Build history of the part. All positions in model axes, mm. Face numbers are marked on the shaded views. A direction names the side the tool comes from. Round coordinates to 2 decimals unless told otherwise and drop trailing zeros. Loops run counter-clockwise (first coordinate to the right, second up) from the corner with the lowest first, then second, coordinate; pieces in that order, holes last.
from build123d import *

# Parameters (mm, degrees)
SKETCH1_R                = 48
SKETCH1_R_2              = 5.25
BOSS_EXTRUDE1_DEPTH      = 9
SKETCH2_R                = 22.5
CUT_EXTRUDE1_DEPTH       = 3.4
SKETCH3_R                = 12
CUT_EXTRUDE2_DEPTH       = 6.6
BOSS_EXTRUDE2_DEPTH      = 17
BOSS_EXTRUDE2_DEPTH_BACK = 17
SKETCH5_R                = 12
CUT_EXTRUDE3_DEPTH       = 4.5
CUT_EXTRUDE3_DEPTH_BACK  = 4.5
CUT_EXTRUDE4_DEPTH       = 12.5
CUT_EXTRUDE4_DEPTH_BACK  = 85.5
SKETCH8_R                = 12
CUT_EXTRUDE5_DEPTH       = 12.5
CUT_EXTRUDE5_DEPTH_BACK  = 85.5


with BuildPart() as part:
    # Sketch1 → Boss-Extrude1 (new body)
    with BuildSketch(Plane(origin=(0, 0, 0), x_dir=(1, 0, 0), z_dir=(0, 1, 0))):
        Circle(SKETCH1_R)
        with Locations((0, 40)):
            Circle(SKETCH1_R_2, mode=Mode.SUBTRACT)
        with Locations((40, 0)):
            Circle(SKETCH1_R_2, mode=Mode.SUBTRACT)
        with Locations((0, -40)):
            Circle(SKETCH1_R_2, mode=Mode.SUBTRACT)
        with Locations((-40, 0)):
            Circle(SKETCH1_R_2, mode=Mode.SUBTRACT)
    extrude(amount=BOSS_EXTRUDE1_DEPTH)

    # Sketch2 → Cut-Extrude1 (cut)
    with BuildSketch(Plane(origin=(0, 9, 0), x_dir=(1, 0, 0), z_dir=(0, 1, 0))):
        Circle(SKETCH2_R)
    extrude(amount=-CUT_EXTRUDE1_DEPTH, mode=Mode.SUBTRACT)

    # Sketch3 → Cut-Extrude2 (cut, through all)
    with BuildSketch(Plane(origin=(0, 5.6, 0), x_dir=(1, 0, 0), z_dir=(0, 1, 0))):
        Circle(SKETCH3_R)
    extrude(amount=-CUT_EXTRUDE2_DEPTH, mode=Mode.SUBTRACT)

    # Sketch4 → Boss-Extrude2 (add, two sides)
    with BuildSketch(Plane.XY) as boss_extrude2_sk:
        with BuildLine():
            Line((-36.5, -66), (-36.5, -32))
            ThreePointArc((-36.5, -32), (-36.207106781, -31.292893219), (-35.5, -31))
            Line((-35.5, -31), (-35.5, -15))
            ThreePointArc((-35.5, -15), (-34.482827555, -7.237912652), (-31.5, 0))
            Line((-31.5, 0), (31.5, 0))
            ThreePointArc((31.5, 0), (34.482827555, -7.237912652), (35.5, -15))
            Line((35.5, -15), (35.5, -31))
            ThreePointArc((35.5, -31), (36.207106781, -31.292893219), (36.5, -32))
            Line((36.5, -32), (36.5, -66))
            ThreePointArc((36.5, -66), (36.207106781, -66.707106781), (35.5, -67))
            Line((35.5, -67), (19.5, -67))
            ThreePointArc((19.5, -67), (18.792893219, -66.707106781), (18.5, -66))
            Line((18.5, -66), (18.5, -12))
            ThreePointArc((18.5, -12), (16.156854249, -6.343145751), (10.5, -4))
            Line((10.5, -4), (-10.5, -4))
            ThreePointArc((-10.5, -4), (-16.156854249, -6.343145751), (-18.5, -12))
            Line((-18.5, -12), (-18.5, -66))
            ThreePointArc((-18.5, -66), (-18.792893219, -66.707106781), (-19.5, -67))
            Line((-19.5, -67), (-35.5, -67))
            ThreePointArc((-35.5, -67), (-36.207106781, -66.707106781), (-36.5, -66))
        make_face()
    extrude(amount=BOSS_EXTRUDE2_DEPTH)
    extrude(boss_extrude2_sk.sketch, amount=-BOSS_EXTRUDE2_DEPTH_BACK)

    # Sketch5 → Cut-Extrude3 (cut, two sides)
    with BuildSketch(Plane.XZ.offset(4)) as cut_extrude3_sk:
        Circle(SKETCH5_R)
    extrude(amount=CUT_EXTRUDE3_DEPTH, mode=Mode.SUBTRACT)
    extrude(cut_extrude3_sk.sketch, amount=-CUT_EXTRUDE3_DEPTH_BACK, mode=Mode.SUBTRACT)

    # Sketch7 → Cut-Extrude4 (cut, two sides)
    with BuildSketch(Plane.ZY.offset(36.5)) as cut_extrude4_sk:
        with BuildLine():
            Line((-17, 0), (-17, -49))
            ThreePointArc((-17, -49), (0, -66), (17, -49))
            Line((17, -49), (17, 0))
            Line((17, 0), (31.554606814, 0))
            Line((31.554606814, 0), (31.554606814, -74.298240475))
            Line((31.554606814, -74.298240475), (-29.742859054, -74.298240475))
            Line((-29.742859054, -74.298240475), (-29.742859054, 0))
            Line((-29.742859054, 0), (-17, 0))
        make_face()
    extrude(amount=CUT_EXTRUDE4_DEPTH, mode=Mode.SUBTRACT)
    extrude(cut_extrude4_sk.sketch, amount=-CUT_EXTRUDE4_DEPTH_BACK, mode=Mode.SUBTRACT)

    # Sketch8 → Cut-Extrude5 (cut, two sides)
    with BuildSketch(Plane(origin=(36.5, 0, 0), x_dir=(0, 0, -1), z_dir=(1, 0, 0))) as cut_extrude5_sk:
        with Locations((0, -49)):
            Circle(SKETCH8_R)
    extrude(amount=CUT_EXTRUDE5_DEPTH, mode=Mode.SUBTRACT)
    extrude(cut_extrude5_sk.sketch, amount=-CUT_EXTRUDE5_DEPTH_BACK, mode=Mode.SUBTRACT)


solid = part.part
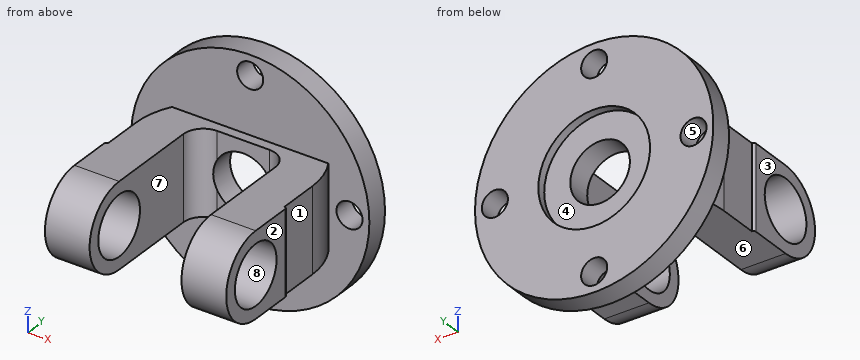
(1) Probe line 1 (X direction, y = 7, z = 0); line 2 (X direction, y = 3.25, z = 0). List the from-to ranges inside material, lowest first.
Responses:
line 1: x = -48 to -45.25, -34.75 to -22.5, 22.5 to 34.75, 45.25 to 48
line 2: x = -48 to -45.25, -34.75 to -12, 12 to 34.75, 45.25 to 48
(2) Which spindle directions (+Z, -Z, +X, -X, +Y, -Y) get a long thin tool onto all of the face, cutting with end or side? Do the marked faces 1, 2, 3 and 4. Say none if no direction does.
Responses:
face 1: +Z, -Z, +X
face 2: +Z, -Z, +X, -Y
face 3: +Z, -Z, -X, -Y
face 4: +Y
(3) Pin check, flat tips, straight feed: P1, Ø3, axis at x = -21.5, y = -47.5, coming from the +Z side; P2, Ø12.5, axis at x = 1.5, z = -13, coming from the -Y side; P3, Ø19, axis at x = 0, z = 0, coming from the +Y side; P4, Ø17.5, axis at y = -20, z = -7.5, coming from the +X side. Stop position of each tip, or through.
Responses:
P1: stops at z = 17
P2: stops at y = -4
P3: passes through
P4: stops at x = 35.5
(4) Slice it at B-B on z = -36.5. List the corners of the cut face in (x, y).
Responses:
outline: (-31.17, 0) - (-3.91, 0) - (-3.91, 9) - (-31.17, 9) - close; (3.91, 0) - (31.17, 0) - (31.17, 9) - (3.91, 9) - close
(5) Slice it at D-D on y = 1.5. List the corners of the cut face in (x, z).
Responses:
outline: circle Ø96 at (0, 0); hole circle Ø10.5 at (-40, 0); hole circle Ø24 at (0, 0); hole circle Ø10.5 at (0, -40); hole circle Ø10.5 at (0, 40); hole circle Ø10.5 at (40, 0)
(6) Pull direction Z, two halves, no side cores. Call the marked faces 5, 6, 7 and 8: +Z half, -Z half, draft (parallel to the pull), parting line (faces both ways), or undercut.
Responses:
face 5: undercut
face 6: -Z half
face 7: draft
face 8: undercut
(7) Slice it at A-A on x = 0. List the corners of the cut face in (y, z).
Responses:
outline: (-4, -17) - (0, -17) - (0, -34.75) - (9, -34.75) - (9, -22.5) - (5.6, -22.5) - (5.6, -12) - (-4, -12) - close; (-4, 12) - (5.6, 12) - (5.6, 22.5) - (9, 22.5) - (9, 34.75) - (0, 34.75) - (0, 17) - (-4, 17) - close; (0, -48) - (9, -48) - (9, -45.25) - (0, -45.25) - close; (0, 45.25) - (9, 45.25) - (9, 48) - (0, 48) - close
(8) Slice it at C-C on x = 40. List the corners of the cut face in (y, z), plus the area to 3 significant figures.
Responses:
outline: (0, -26.53) - (9, -26.53) - (9, -5.25) - (0, -5.25) - close; (0, 5.25) - (9, 5.25) - (9, 26.53) - (0, 26.53) - close
area: 383 mm2
